```python
from build123d import *

# Parameters (mm, degrees)
BOSS_EXTRUDE1_DEPTH                                = 12.5
SKETCH2_W                                          = 2
SKETCH2_H                                          = 26
CUT_EXTRUDE1_DEPTH                                 = 43
SKETCH3_W                                          = 26
SKETCH3_H                                          = 2
CUT_EXTRUDE2_DEPTH                                 = 43
SKETCH4_R                                          = 3.25
CUT_EXTRUDE3_DEPTH                                 = 3
SKETCH5_R                                          = 2.5
CUT_EXTRUDE4_DEPTH                                 = 11.5
CBORE_FOR_M2_5_PAN_HEAD_MACHINE_SCREW1_D           = 2.9
CBORE_FOR_M2_5_PAN_HEAD_MACHINE_SCREW1_CBORE_D     = 6
CBORE_FOR_M2_5_PAN_HEAD_MACHINE_SCREW1_CBORE_DEPTH = 2.1
FILLET1_R                                          = 2


with BuildPart() as part:
    # Sketch1 → Boss-Extrude1 (new body)
    with BuildSketch(Plane.XY):
        Polygon((-17.465670258, 21), (-21, 17.012864847), (-21, -17.012864847), (-17.465670258, -21), (17.465670258, -21), (21, -17.012864847), (21, 17.012864847), (17.465670258, 21), align=None)
    extrude(amount=BOSS_EXTRUDE1_DEPTH)

    # Sketch2 → Cut-Extrude1 (cut, through all)
    with BuildSketch(Plane(origin=(21, 0, 0), x_dir=(0, 0, -1), z_dir=(1, 0, 0))):
        with Locations((-11.5, 0)):
            Rectangle(SKETCH2_W, SKETCH2_H)
    extrude(amount=-CUT_EXTRUDE1_DEPTH, mode=Mode.SUBTRACT)

    # Sketch3 → Cut-Extrude2 (cut, through all)
    with BuildSketch(Plane.XZ.offset(21)):
        with Locations((0, 11.5)):
            Rectangle(SKETCH3_W, SKETCH3_H)
    extrude(amount=-CUT_EXTRUDE2_DEPTH, mode=Mode.SUBTRACT)

    # Sketch4 → Cut-Extrude3 (cut)
    with BuildSketch(Plane(origin=(0, 0, 0), x_dir=(-1, 0, 0), z_dir=(0, 0, -1))):
        Circle(SKETCH4_R)
    extrude(amount=-CUT_EXTRUDE3_DEPTH, mode=Mode.SUBTRACT)

    # Sketch5 → Cut-Extrude4 (cut, through all)
    with BuildSketch(Plane.XY.offset(10.5)):
        Circle(SKETCH5_R)
    extrude(amount=-CUT_EXTRUDE4_DEPTH, mode=Mode.SUBTRACT)

    # CBORE for M2.5 Pan Head Machine Screw1 (through all)
    with Locations(Plane(origin=(0, 0, 0), x_dir=(-1, 0, 0), z_dir=(0, 0, -1))):
        with Locations((-15.5, 15.5), (15.5, 15.5), (15.5, -15.5), (-15.5, -15.5)):
            CounterBoreHole(CBORE_FOR_M2_5_PAN_HEAD_MACHINE_SCREW1_D / 2, CBORE_FOR_M2_5_PAN_HEAD_MACHINE_SCREW1_CBORE_D / 2, CBORE_FOR_M2_5_PAN_HEAD_MACHINE_SCREW1_CBORE_DEPTH)

    # Fillet1
    fillet1_edges = [part.edges().sort_by_distance(p)[0] for p in [
        (17.465670258, 21, 6.25),
        (21, 17.012864847, 6.25),
        (21, -17.012864847, 6.25),
        (17.465670258, -21, 6.25),
        (-17.465670258, -21, 6.25),
        (-21, -17.012864847, 6.25),
        (-21, 17.012864847, 6.25),
        (-17.465670258, 21, 6.25),
    ]]
    fillet(fillet1_edges, radius=FILLET1_R)


solid = part.part
```
CAD build for the part. Positions are in the model's coordinates, mm. A direction names the side the tool comes from. Round coordinates to 2 decimals unless told otherwise and drop trailing zeros. Write each loop counter-clockwise with the first axis right and the second up, starting at its lowest first coordinate (ties: lowest second). Pieces come first, ordered by that corner, then holes. Notation, with made-up numbers: (58.25, -36.5) - (70.25, -36.5) arc R24 ccw to (70.25, -17.5) - close; hole circle Ø3 at (83.25, -34). An arc over 180 degrees is marked (long way). Return JSON: item names as keys, results as strings. Group by question number.
Item 1: Probe probe 1 along Y at (x, z) = (-15.5, 6.5); probe 2 along Y at (x, z) = (15.5, 1.3); probe 3 along Y at (x, z) = (0, 6.25). List the from-to ranges inside material, lowest first.
Item 2: Band-saw the part on C-C on z = 6.5. List the corners of the cut face in (x, y).
Item 3: Flat gauge pins, fed straight in: pin 1 Ø4 at (x, y) = (15.5, -15.5) entering from -Z; pin 2 Ø0.6 at (x, z) = (18, 11.5) entering from +Y; pin 3 Ø2 at (x, y) = (1.5, 0.5) entering from -Z. Where does each tip first touch, or does it go through?
Item 4: Band-saw the part on D-D on x = 15.5. List the corners of the cut face in (y, z), plus the area to 3 significant figures.
Item 5: Band-saw the part on A-A on y = 0. List the corners of the cut face in (x, z).
Item 6: 3-axis set-ups, long thin cutter, end or side, ignore diameter. For faces 1 (the face through (-13, -17, 11)), 2 (the face through (17.376, 20.829, 6.338)), 3 (the face through (-17, 13, 12)): which of +Z, -Z, +X, -X, +Y, -Y reach the whole face in a straight line?
Item 7: Mould opens along X. For faces 4 (the face through (17, 17, 12.5)), 5 (the face through (16.88, 15.94, 7.37)), 6 (the face through (20.866, 16.973, 6.338)) say: +X half, -X half, draft (parallel to the pull), parting line (faces both ways), or undercut.
Resolved:
{
 "1": {"probe 1": "y = -21 to -16.95, -14.05 to 14.05, 16.95 to 21", "probe 2": "y = -21 to -18.5, -12.5 to 12.5, 18.5 to 21", "probe 3": "y = -21 to -2.5, 2.5 to 21"},
 "2": {"outline": "(-21, -16.25) arc R2 ccw to (-20.5, -17.58) - (-18.06, -20.33) arc R2 ccw to (-16.57, -21) - (16.57, -21) arc R2 ccw to (18.06, -20.33) - (20.5, -17.58) arc R2 ccw to (21, -16.25) - (21, 16.25) arc R2 ccw to (20.5, 17.58) - (18.06, 20.33) arc R2 ccw to (16.57, 21) - (-16.57, 21) arc R2 ccw to (-18.06, 20.33) - (-20.5, 17.58) arc R2 ccw to (-21, 16.25) - close; hole circle Ø2.9 at (-15.5, -15.5); hole circle Ø2.9 at (-15.5, 15.5); hole circle Ø5 at (0, 0); hole circle Ø2.9 at (15.5, -15.5); hole circle Ø2.9 at (15.5, 15.5)"},
 "3": {"pin 1": "stops at z = 2.1", "pin 2": "stops at y = 20.65", "pin 3": "stops at z = 3"},
 "4": {"outline": "(-21, 0) - (-18.5, 0) - (-18.5, 2.1) - (-16.95, 2.1) - (-16.95, 12.5) - (-21, 12.5) - close; (-14.05, 2.1) - (-12.5, 2.1) - (-12.5, 0) - (12.5, 0) - (12.5, 2.1) - (14.05, 2.1) - (14.05, 12.5) - (13, 12.5) - (13, 10.5) - (-13, 10.5) - (-13, 12.5) - (-14.05, 12.5) - close; (16.95, 2.1) - (18.5, 2.1) - (18.5, 0) - (21, 0) - (21, 12.5) - (16.95, 12.5) - close", "area": "387 mm²"},
 "5": {"outline": "(-21, 0) - (-3.25, 0) - (-3.25, 3) - (-2.5, 3) - (-2.5, 10.5) - (-21, 10.5) - close; (2.5, 3) - (3.25, 3) - (3.25, 0) - (21, 0) - (21, 10.5) - (2.5, 10.5) - close"},
 "6": {"face 1": "+Z, +Y, -Y", "face 2": "+Z, -Z, +X, +Y", "face 3": "+Z, +X, -X"},
 "7": {"face 4": "draft", "face 5": "undercut", "face 6": "+X half"}
}
